CAD build for the part. Positions are in the model's coordinates, mm. Face numbers are marked on the shaded views. A direction names the side the tool comes from. Round coordinates to 2 decimals unless told otherwise and drop trailing zeros. Write each loop counter-clockwise with the first axis right and the second up, starting at its lowest first coordinate (ties: lowest second). Pieces come first, ordered by that corner, then holes. Notation, with made-up numbers: M 68,50 L 92,50 A23 ccw 92,76 Z; hole C 26.25,-19 d8. An arc over 180 degrees is marked long. Write each question's results on one line, items separated by ' | '. Start each with the question number.
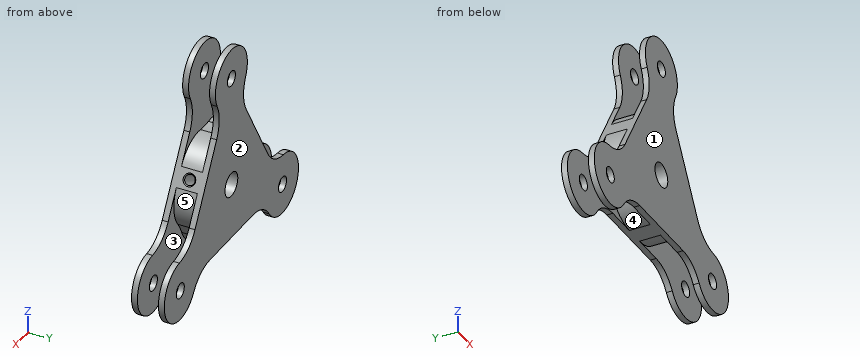
```python
from build123d import *

# Parameters (mm, degrees)
ESQUISSE1_R             = 12.5
ESQUISSE1_R_2           = 5
BOSS_EXTRU_1_DEPTH      = 6.75
ESQUISSE7_R             = 24
ENL_V_MAT_EXTRU_1_DEPTH = 4.325
CONG_6_START            = -4.325
CONG_6_DEPTH            = 8.65
CONG_7_R                = 15
ESQUISSE25_R            = 3.15
ENL_V_MAT_EXTRU_2_DEPTH = 80.892326756


with BuildPart() as part:
    # Esquisse1 → Boss.-Extru.1 (new, symmetric)
    # profile 1 of 16: a face of its own
    with BuildSketch(Plane(origin=(0, 0, 0), x_dir=(1, 0, 0), z_dir=(0, 1, 0))):
        with Locations((-40, 23.094010768)):
            Circle(ESQUISSE1_R)
    # profile 2 of 16: a face of its own
    with BuildSketch(Plane(origin=(0, 0, 0), x_dir=(1, 0, 0), z_dir=(0, 1, 0))):
        with Locations((0, -46.188021535)):
            Circle(ESQUISSE1_R)
    # profile 3 of 16: a face of its own
    with BuildSketch(Plane(origin=(0, 0, 0), x_dir=(1, 0, 0), z_dir=(0, 1, 0))):
        with Locations((40, 23.094010768)):
            Circle(ESQUISSE1_R)
    # profile 4 of 16: a face of its own
    with BuildSketch(Plane(origin=(0, 0, 0), x_dir=(1, 0, 0), z_dir=(0, 1, 0))):
        Polygon((0, -46.188021535), (-40, 23.094010768), (40, 23.094010768), align=None)
        with Locations(Location((0, 0, 0), (0, 0, 270))):
            Circle(ESQUISSE1_R_2, mode=Mode.SUBTRACT)
    # profile 5 of 16: a face of its own
    with BuildSketch(Plane(origin=(0, 0, 0), x_dir=(1, 0, 0), z_dir=(0, 1, 0))):
        with BuildLine():
            ThreePointArc((-33.75, 12.26869322), (-29.174682453, 16.844010768), (-27.5, 23.094010768))
            Line((-27.5, 23.094010768), (-40, 23.094010768))
            Line((-40, 23.094010768), (-33.75, 12.26869322))
        make_face()
    # profile 6 of 16: a face of its own
    with BuildSketch(Plane(origin=(0, 0, 0), x_dir=(1, 0, 0), z_dir=(0, 1, 0))):
        with BuildLine():
            Line((-40, 23.094010768), (-27.5, 23.094010768))
            ThreePointArc((-27.5, 23.094010768), (-50.825317547, 29.344010768), (-33.75, 12.26869322))
            Line((-33.75, 12.26869322), (-40, 23.094010768))
        make_face()
    # profile 7 of 16: a face of its own
    with BuildSketch(Plane(origin=(0, 0, 0), x_dir=(1, 0, 0), z_dir=(0, 1, 0))):
        with BuildLine():
            Line((27.5, 23.094010768), (40, 23.094010768))
            Line((40, 23.094010768), (33.75, 12.26869322))
            ThreePointArc((33.75, 12.26869322), (46.25, 12.26869322), (52.5, 23.094010768))
            ThreePointArc((52.5, 23.094010768), (40, 35.594010768), (27.5, 23.094010768))
        make_face()
    # profile 8 of 16: a face of its own
    with BuildSketch(Plane(origin=(0, 0, 0), x_dir=(1, 0, 0), z_dir=(0, 1, 0))):
        with BuildLine():
            Line((33.75, 12.26869322), (40, 23.094010768))
            Line((40, 23.094010768), (27.5, 23.094010768))
            ThreePointArc((27.5, 23.094010768), (29.174682453, 16.844010768), (33.75, 12.26869322))
        make_face()
    # profile 9 of 16: a face of its own
    with BuildSketch(Plane(origin=(0, 0, 0), x_dir=(1, 0, 0), z_dir=(0, 1, 0))):
        with BuildLine():
            Line((27.5, 23.094010768), (40, 23.094010768))
            Line((40, 23.094010768), (33.75, 12.26869322))
            ThreePointArc((33.75, 12.26869322), (46.25, 12.26869322), (52.5, 23.094010768))
            ThreePointArc((52.5, 23.094010768), (40, 35.594010768), (27.5, 23.094010768))
        make_face()
    # profile 10 of 16: a face of its own
    with BuildSketch(Plane(origin=(0, 0, 0), x_dir=(1, 0, 0), z_dir=(0, 1, 0))):
        with BuildLine():
            Line((33.75, 12.26869322), (40, 23.094010768))
            Line((40, 23.094010768), (27.5, 23.094010768))
            ThreePointArc((27.5, 23.094010768), (29.174682453, 16.844010768), (33.75, 12.26869322))
        make_face()
    # profile 11 of 16: a face of its own
    with BuildSketch(Plane(origin=(0, 0, 0), x_dir=(1, 0, 0), z_dir=(0, 1, 0))):
        with BuildLine():
            ThreePointArc((-33.75, 12.26869322), (-29.174682453, 16.844010768), (-27.5, 23.094010768))
            Line((-27.5, 23.094010768), (-40, 23.094010768))
            Line((-40, 23.094010768), (-33.75, 12.26869322))
        make_face()
    # profile 12 of 16: a face of its own
    with BuildSketch(Plane(origin=(0, 0, 0), x_dir=(1, 0, 0), z_dir=(0, 1, 0))):
        with BuildLine():
            Line((-40, 23.094010768), (-27.5, 23.094010768))
            ThreePointArc((-27.5, 23.094010768), (-50.825317547, 29.344010768), (-33.75, 12.26869322))
            Line((-33.75, 12.26869322), (-40, 23.094010768))
        make_face()
    # profile 13 of 16: a face of its own
    with BuildSketch(Plane(origin=(0, 0, 0), x_dir=(1, 0, 0), z_dir=(0, 1, 0))):
        with BuildLine():
            ThreePointArc((12.5, -46.188021535), (10.825317547, -39.938021535), (6.25, -35.362703988))
            Line((6.25, -35.362703988), (0, -46.188021535))
            Line((0, -46.188021535), (-6.25, -35.362703988))
            ThreePointArc((-6.25, -35.362703988), (-6.25, -57.013339082), (12.5, -46.188021535))
        make_face()
    # profile 14 of 16: a face of its own
    with BuildSketch(Plane(origin=(0, 0, 0), x_dir=(1, 0, 0), z_dir=(0, 1, 0))):
        with BuildLine():
            Line((0, -46.188021535), (6.25, -35.362703988))
            ThreePointArc((6.25, -35.362703988), (0, -33.688021535), (-6.25, -35.362703988))
            Line((-6.25, -35.362703988), (0, -46.188021535))
        make_face()
    # profile 15 of 16: a face of its own
    with BuildSketch(Plane(origin=(0, 0, 0), x_dir=(1, 0, 0), z_dir=(0, 1, 0))):
        with BuildLine():
            ThreePointArc((12.5, -46.188021535), (10.825317547, -39.938021535), (6.25, -35.362703988))
            Line((6.25, -35.362703988), (0, -46.188021535))
            Line((0, -46.188021535), (-6.25, -35.362703988))
            ThreePointArc((-6.25, -35.362703988), (-6.25, -57.013339082), (12.5, -46.188021535))
        make_face()
    # profile 16 of 16: a face of its own
    with BuildSketch(Plane(origin=(0, 0, 0), x_dir=(1, 0, 0), z_dir=(0, 1, 0))):
        with BuildLine():
            Line((0, -46.188021535), (6.25, -35.362703988))
            ThreePointArc((6.25, -35.362703988), (0, -33.688021535), (-6.25, -35.362703988))
            Line((-6.25, -35.362703988), (0, -46.188021535))
        make_face()
    extrude(amount=BOSS_EXTRU_1_DEPTH, both=True)

    # Esquisse7 → Enlèv. mat.-Extru.1 (cut, symmetric)
    with BuildSketch(Plane(origin=(0, 0, 0), x_dir=(1, 0, 0), z_dir=(0, 1, 0))):
        with Locations((-40, 23.094010768)):
            Circle(ESQUISSE7_R)
        with Locations((0, -46.188021535)):
            Circle(ESQUISSE7_R)
        with Locations((40, 23.094010768)):
            Circle(ESQUISSE7_R)
    extrude(amount=ENL_V_MAT_EXTRU_1_DEPTH, both=True, mode=Mode.SUBTRACT)

    # Congé6: read off the stored shape, not the designer's step
    # Congé6 outline → Congé6 (cut)
    with BuildSketch(Plane(origin=(0, 0, 0), x_dir=(1, 0, 0), z_dir=(0, 1, 0)).offset(CONG_6_START)):
        with BuildLine():
            ThreePointArc((4, 23.094010768), (12.320502943, 20.574765183), (17.846153846, 13.863241537))
            ThreePointArc((17.846153846, 13.863241537), (16.466063783, 18.387223525), (16, 23.094010768))
            Line((16, 23.094010768), (4, 23.094010768))
        make_face()
        with BuildLine():
            ThreePointArc((28, 2.309401077), (24.156834569, 5.066417775), (20.928996273, 8.523601822))
            ThreePointArc((20.928996273, 8.523601822), (23.978520797, 0.382485945), (22, -8.082903769))
            Line((22, -8.082903769), (28, 2.309401077))
        make_face()
        with BuildLine():
            ThreePointArc((-17.846153846, 13.863241537), (-12.320502943, 20.574765183), (-4, 23.094010768))
            Line((-4, 23.094010768), (-16, 23.094010768))
            ThreePointArc((-16, 23.094010768), (-16.466063783, 18.387223525), (-17.846153846, 13.863241537))
        make_face()
        with BuildLine():
            Line((12, -25.403411844), (18, -15.011106999))
            ThreePointArc((18, -15.011106999), (11.658017854, -20.957251128), (3.082842427, -22.386843359))
            ThreePointArc((3.082842427, -22.386843359), (7.690770786, -23.453641299), (12, -25.403411844))
        make_face()
        with BuildLine():
            ThreePointArc((-22, -8.082903769), (-23.978520797, 0.382485945), (-20.928996273, 8.523601822))
            ThreePointArc((-20.928996273, 8.523601822), (-24.156834569, 5.066417775), (-28, 2.309401077))
            Line((-28, 2.309401077), (-22, -8.082903769))
        make_face()
        with BuildLine():
            ThreePointArc((-12, -25.403411844), (-7.690770786, -23.453641299), (-3.082842427, -22.386843359))
            ThreePointArc((-3.082842427, -22.386843359), (-11.658017854, -20.957251128), (-18, -15.011106999))
            Line((-18, -15.011106999), (-12, -25.403411844))
        make_face()
    extrude(amount=CONG_6_DEPTH, mode=Mode.SUBTRACT)

    # Trou taraudé M51: read off the stored shape, not the designer's step
    # Trou taraudé M51 outline → Trou taraudé M51 (revolve, cut)
    with BuildSketch(Plane(origin=(0, 0, 0), x_dir=(0.5000000000000003, 0, -0.8660254037844385), z_dir=(0, -1, 0))):
        Polygon((0, 4.537411543), (2.1, 4.537411543), (2.1, 22.669010768), (2.525, 23.094010768), (0, 23.094010768), align=None)
    revolve(axis=Axis((0, 0, 0), (0.8660254037844385, 0, 0.5000000000000003)), mode=Mode.SUBTRACT)

    # Congé7
    cong_7_edges = [part.edges().sort_by_distance(p)[0] for p in [
        (-27.5, 5.5375, -23.094010768),
        (27.5, 5.5375, -23.094010768),
        (33.75, 5.5375, -12.26869322),
        (6.25, 5.5375, 35.362703988),
        (-6.25, 5.5375, 35.362703988),
        (-33.75, 5.5375, -12.26869322),
        (-27.5, -5.5375, -23.094010768),
        (27.5, -5.5375, -23.094010768),
        (33.75, -5.5375, -12.26869322),
        (6.25, -5.5375, 35.362703988),
        (-6.25, -5.5375, 35.362703988),
        (-33.75, -5.5375, -12.26869322),
    ]]
    fillet(cong_7_edges, radius=CONG_7_R)

    # Esquisse25 → Enlèv. mat.-Extru.2 (cut, through all)
    with BuildSketch(Plane(origin=(0, 6.75, 0), x_dir=(1, 0, 0), z_dir=(0, 1, 0))):
        with Locations(Location((-40, 23.094010768, 0), (0, 0, 270))):
            Circle(ESQUISSE25_R)
        with Locations(Location((40, 23.094010768, 0), (0, 0, 270))):
            Circle(ESQUISSE25_R)
        with Locations(Location((0, -46.188021535, 0), (0, 0, 270))):
            Circle(ESQUISSE25_R)
    extrude(amount=-ENL_V_MAT_EXTRU_2_DEPTH, mode=Mode.SUBTRACT)


solid = part.part
```
1) Saw through at B-B, the plane x = 35.5. Write the cut outline in (y, z) (3 decimals), plus the area to 3 significant figures.
2) 3-axis set-ups, long thin cutter, end or side, ignore diameter. For the marked faces 4 and 5: which of +Z, -Z, +X, -X, +Y, -Y reach the whole face in a straight line?
3) Wall check: line 1 along Y through (x, z) = (3.5, 46.5) (3 decimals); line 2 along X through (y, z) = (-3.25, 0); line 3 along X through (y, z) = (5, -24.5). Give the ranges that are in metal, low to high. Write a range as from..to.
4) Pull direction Y, two halves, no side cores. Call the marked faces 1, 2 and 3: pulls with the +Y half, pulls with the -Y half, needs draft (parallel to the pull), parting line crosses it, or undercut.
5) Saw through at C-C, the plane x = -42. Write the cut outline in (y, z) (3 decimals).
6) Drop flat-ended pins along their axis: pin 1 Ø1 at (y, z) = (2, 16.5) entering from -X; pin 2 Ø8 at (x, y) = (25, -3.5) entering from -Z; pin 3 Ø1 at (y, z) = (-1, 9) entering from -X. Give the stop position or say it passes through.
7) Saw through at A-A, the plane z = -25. State how many separate pieces and enclosed holes the cut face has, plus the area to 3 significant figures.
Filled sheet:
1) outline: M -6.75,-34.756 L -4.325,-34.756 L -4.325,-9.396 L -6.75,-9.396 Z; M 4.325,-34.756 L 6.75,-34.756 L 6.75,-9.396 L 4.325,-9.396 Z | area: 123 mm^2
2) face 4: -Z, -X | face 5: +X
3) line 1: y = -6.75..-4.325, 4.325..6.75 | line 2: x = -24..-5, 5..24 | line 3: x = -52.42..-42.82, -37.18..-23.29, 23.29..37.18, 42.82..52.42
4) face 1: pulls with the -Y half | face 2: pulls with the +Y half | face 3: undercut
5) outline: M -6.75,-35.433 L -4.325,-35.433 L -4.325,-25.528 L -6.75,-25.528 Z; M -6.75,-20.66 L -4.325,-20.66 L -4.325,-10.755 L -6.75,-10.755 Z; M 4.325,-35.433 L 6.75,-35.433 L 6.75,-25.528 L 4.325,-25.528 Z; M 4.325,-20.66 L 6.75,-20.66 L 6.75,-10.755 L 4.325,-10.755 Z
6) pin 1: stops at x = -17.38 | pin 2: stops at z = -29.04 | pin 3: stops at x = -21.76
7) separate pieces: 8 | enclosed holes: 0 | area: 224 mm^2
